from build123d import *

# Parameters (mm, degrees)
SKETCH1_W           = 16.5
SKETCH1_H           = 58.5
BOSS_EXTRUDE1_DEPTH = 16.5
SKETCH4_R           = 1.77
BOSS_EXTRUDE6_DEPTH = 1
SKETCH4_16_R        = 4.05


with BuildPart() as part:
    # Sketch1 → Boss-Extrude1 (new body)
    with BuildSketch(Plane.XY):
        Rectangle(SKETCH1_W, SKETCH1_H)
    extrude(amount=BOSS_EXTRUDE1_DEPTH)

    # Sketch4 → Boss-Extrude6 (add)
    with BuildSketch(Plane.XY.offset(16.5)):
        with Locations(Location((0, 0, 0), (0, 0, 180))):
            Circle(SKETCH4_R)
    extrude(amount=BOSS_EXTRUDE6_DEPTH)

    # Sketch4_16 → section 0 of loft3
    with BuildSketch(Plane.XY.offset(16.5), mode=Mode.PRIVATE) as loft3_s0:
        Circle(SKETCH4_16_R)
    # loft up to a face of the part (loft3)
    loft([loft3_s0.sketch, Face(Wire([part.edges().sort_by_distance((1.211648377, -1.290274471, 17.5))[0]]))])


solid = part.part
Geometry check sheet. Reference: the model listing, model coordinates, mm. Coordinates: 2 decimals unless noted, no trailing zeros. Order: outer loops, then holes, each group sorted by start corner. A loop starts at its lowest first (then second) coordinate and runs counter-clockwise, first axis right, second up. Notation, with made-up numbers: (26.25, 46) - (33.25, 46) arc R22 cw to (33.25, 84) - close; hole circle Ø8 at (64.5, 36.25). An arc over 180 degrees is marked (long way). Answer in a Markdown table with one row per item. Add a question column.
1) Cross-section at A-A, the plane x = 0. Record the cut outline in (y, z).
2) Material ranges on line 1 along Z through (x, y) = (0.5, -10.5); line 2 along Z through (x, y) = (-1.5, -1), recorded low to high. Write a range as [from, to].
3) Cross-section at B-B, the plane y = -13.5. Record the cut outline in (x, z), then the cut area to 3 significant figures.
4) Gauge pin test, flat end, axial feed: P1, Ø5, axis at x = 0, y = 9.5, coming from the -Z side. Record the tip position at first contact, or that the pin passes through.
5) Cross-section at C-C, the plane x = 5.5. Record the cut outline in (y, z), then the cut area to 3 significant figures.
Check result:
| question | item | result |
|---|---|---|
| 1 | outline | (-29.25, 0) - (29.25, 0) - (29.25, 16.5) - (4.05, 16.5) - (1.77, 17.5) - (-1.77, 17.5) - (-4.05, 16.5) - (-29.25, 16.5) - close |
| 2 | line 1 | z = [0, 16.5] |
| 2 | line 2 | z = [0, 17.49] |
| 3 | outline | (-8.25, 0) - (8.25, 0) - (8.25, 16.5) - (-8.25, 16.5) - close |
| 3 | area | 272 mm² |
| 4 | P1 | stops at z = 0 |
| 5 | outline | (-29.25, 0) - (29.25, 0) - (29.25, 16.5) - (-29.25, 16.5) - close |
| 5 | area | 965 mm² |
